Work out the finished part from the listing and answer in its coordinate system (mm). A direction names the side the tool comes from. Round coordinates to 2 decimals unless told otherwise and drop trailing zeros. Order: outer loops, then holes, each group sorted by start corner. A loop starts at its lowest first (then second) coordinate and runs counter-clockwise, first axis right, second up.
from build123d import *

# Parameters (mm, degrees)
SKETCH_W        = 150
SKETCH_H        = 30
PAD_DEPTH       = 5
SKETCH001_W     = 150
SKETCH001_H     = 5
PAD001_DEPTH    = 40
SKETCH002_R     = 14.5
SKETCH002_R_2   = 7.75
POCKET_DEPTH    = 30.001
FILLET_R        = 10
SKETCH003_W     = 10
SKETCH003_H     = 6
PAD002_DEPTH    = 3
SKETCH005_W     = 5
SKETCH005_H     = 20
PAD003_DEPTH    = 20
CHAMFER_SIZE    = 19
SKETCH006_R     = 3
POCKET001_DEPTH = 45.001


with BuildPart() as part:
    # Sketch → Pad (new body)
    with BuildSketch(Plane.XY):
        with Locations((75, 15)):
            Rectangle(SKETCH_W, SKETCH_H)
    extrude(amount=PAD_DEPTH)

    # Sketch001 (on Face6 of Pad) → Pad001 (join)
    with BuildSketch(Plane.XY.offset(5)):
        with Locations((75, 2.5)):
            Rectangle(SKETCH001_W, SKETCH001_H)
    extrude(amount=PAD001_DEPTH)

    # Sketch002 (on Face5 of Pad001) → Pocket (cut, through all)
    with BuildSketch(Plane.XZ):
        with Locations((20, 25)):
            Circle(SKETCH002_R)
        with Locations((75, 25)):
            Circle(SKETCH002_R)
        with Locations((130, 25)):
            Circle(SKETCH002_R_2)
    extrude(amount=-POCKET_DEPTH, mode=Mode.SUBTRACT)

    # Fillet
    fillet_edges = [part.edges().sort_by_distance(p)[0] for p in [
        (150, 2.5, 45),
        (0, 2.5, 45),
    ]]
    fillet(fillet_edges, radius=FILLET_R)

    # Sketch003 → Pad002 (join)
    with BuildSketch(Plane(origin=(0, 0, 0), x_dir=(1, 0, 0), z_dir=(0, 0, -1))):
        with Locations((35, -15)):
            Rectangle(SKETCH003_W, SKETCH003_H)
        with Locations((115, -15)):
            Rectangle(SKETCH003_W, SKETCH003_H)
    extrude(amount=PAD002_DEPTH)

    # Sketch005 → Pad003 (join)
    with BuildSketch(Plane.XY.offset(5)):
        with Locations((47.5, 15)):
            Rectangle(SKETCH005_W, SKETCH005_H)
        with Locations((107.5, 15)):
            Rectangle(SKETCH005_W, SKETCH005_H)
    extrude(amount=PAD003_DEPTH)

    # Chamfer
    chamfer_edges = [part.edges().sort_by_distance(p)[0] for p in [
        (107.5, 25, 25),
        (47.5, 25, 25),
    ]]
    chamfer(chamfer_edges, length=CHAMFER_SIZE)

    # Sketch006 (on Face23 of Chamfer) → Pocket001 (cut, through all)
    with BuildSketch(Plane(origin=(0, 0, 0), x_dir=(1, 0, 0), z_dir=(0, 0, -1))):
        with Locations((10, -15)):
            Circle(SKETCH006_R)
        with Locations((140, -15)):
            Circle(SKETCH006_R)
    extrude(amount=-POCKET001_DEPTH, mode=Mode.SUBTRACT)


solid = part.part
Item 1: Find section A-A (x = 20). Write down the section's boundary in (y, z), plus the area to 3 significant figures.
Item 2: Find section B-B (z = 30.5). Write down the section's boundary in (x, y).
Item 3: A tool of negligible diameter and unlimited length cuts with its end or side. For faces 1 (the face through (115, 18, -1)), 2 (the face through (110, 13, 13)), 3 (the face through (35, 12, -1)), 4 (the face through (50, 13, 13)), from which of +Z, -Z, +X, -X, +Y, -Y can it reach the whole face along a straight path? Write none if from no direction.
Item 4: Find the intervals of material crossed by line 1 along X through (y, z) = (15, 1.85); line 2 along Z through (x, y) = (75, 1.2); line 3 along X through (y, z) = (15.25, 15.5), in increasing order.
Item 5: For a pull along Y with two mould halves and no side action, classify faces 5 (the face through (74, 30, 2)), 6 (the face through (142.77, 16.15, 2.46)), 7 (the face through (74, 3, 45)) as released by +Y, released by -Y, zero draft, split by the parting line, or undercut.
Item 6: Given pin 1 (10 mm diameter, centred on x = 43, y = 4, fed in from -Z); pin 2 (10 mm diameter, centred on x = 76, y = 25, fed in from +Z); pin 3 (18 mm diameter, centred on x = 130, z = 25, fed in from +Y); pin 4 (17.5 mm diameter, centred on x = 75, z = 25, fed in from -Y), each flat-ended and moving along its own axis, determine where each tip first touches the part or whether it passes through.
Item 7: Find section C-C (y = 10). Write down the section's boundary in (x, z).
Item 8: Find section D-D (x = 94). Write down the section's boundary in (y, z).
Model answer:
1. outline: (0, 0) - (30, 0) - (30, 5) - (5, 5) - (5, 10.5) - (0, 10.5) - close; (0, 39.5) - (5, 39.5) - (5, 45) - (0, 45) - close
1. area: 205 mm2
2. outline: (0, 0) - (6.58, 0) - (6.58, 5) - (0, 5) - close; (33.42, 0) - (61.58, 0) - (61.58, 5) - (33.42, 5) - close; (88.42, 0) - (124.54, 0) - (124.54, 5) - (88.42, 5) - close; (135.46, 0) - (150, 0) - (150, 5) - (135.46, 5) - close
3. face 1: -Z, +X, -X, +Y
3. face 2: +Z, +X, +Y
3. face 3: -Z, +X, -X, -Y
3. face 4: +Z, +Y
4. line 1: x = 0 to 7, 13 to 137, 143 to 150
4. line 2: z = 0 to 10.5, 39.5 to 45
4. line 3: x = 45 to 50, 105 to 110
5. face 5: released by +Y
5. face 6: undercut
5. face 7: zero draft
6. pin 1: stops at z = 0
6. pin 2: stops at z = 5
6. pin 3: stops at y = 5
6. pin 4: passes through
7. outline: (0, 0) - (150, 0) - (150, 5) - (110, 5) - (110, 21) - (105, 21) - (105, 5) - (50, 5) - (50, 21) - (45, 21) - (45, 5) - (0, 5) - close
8. outline: (0, 0) - (30, 0) - (30, 5) - (5, 5) - (5, 45) - (0, 45) - close
